The listing builds one solid part. Answer for the finished solid, in the listing's coordinates (mm). Face numbers are marked on the shaded views. A direction names the side the tool comes from. Give positions to 0.01 mm unless a question says otherwise; leave off trailing zeros. Write each loop counter-clockwise with the first axis right and the second up, starting at its lowest first coordinate (ties: lowest second). Pieces come first, ordered by that corner, then holes.
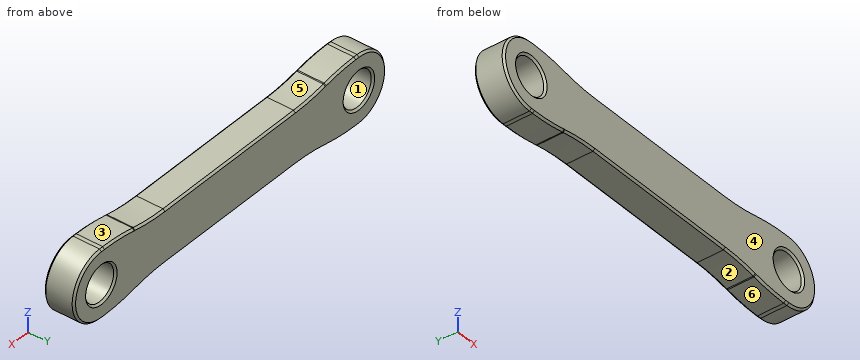
```python
from build123d import *

# Parameters (mm, degrees)
SKETCH1_R           = 4.7
BOSS_EXTRUDE1_DEPTH = 8
FILLET1_R           = 50
FILLET2_R           = 50
CHAMFER1_SIZE       = 0.5
CHAMFER2_SIZE       = 0.5


with BuildPart() as part:
    # Sketch1 → Boss-Extrude1 (new body)
    with BuildSketch(Plane(origin=(0, 0, 0), x_dir=(1, 0, 0), z_dir=(0, 1, 0))):
        with BuildLine():
            Line((6, 9), (16, 7))
            Line((16, 7), (69, 7))
            Line((69, 7), (79, 9))
            Line((79, 9), (85, 9))
            ThreePointArc((85, 9), (94, 0), (85, -9))
            Line((85, -9), (79, -9))
            Line((79, -9), (69, -7))
            Line((69, -7), (16, -7))
            Line((16, -7), (6, -9))
            Line((6, -9), (0, -9))
            ThreePointArc((0, -9), (-9, 0), (0, 9))
            Line((0, 9), (6, 9))
        make_face()
        with Locations(Location((0, 0, 0), (0, 0, 270))):
            Circle(SKETCH1_R, mode=Mode.SUBTRACT)
        with Locations(Location((85, 0, 0), (0, 0, 270))):
            Circle(SKETCH1_R, mode=Mode.SUBTRACT)
    extrude(amount=BOSS_EXTRUDE1_DEPTH)

    # Fillet1
    fillet1_edges = [part.edges().sort_by_distance(p)[0] for p in [
        (16, 4, -7),
        (69, 4, -7),
        (69, 4, 7),
        (16, 4, 7),
    ]]
    fillet(fillet1_edges, radius=FILLET1_R)

    # Fillet2
    fillet2_edges = [part.edges().sort_by_distance(p)[0] for p in [
        (6, 4, 9),
        (6, 4, -9),
        (79, 4, -9),
        (79, 4, 9),
    ]]
    fillet(fillet2_edges, radius=FILLET2_R)

    # Chamfer1
    chamfer1_edges = [part.edges().sort_by_distance(p)[0] for p in [
        (0, 0, -4.7),
        (0, 8, -4.7),
        (85, 0, -4.7),
        (85, 8, -4.7),
    ]]
    chamfer(chamfer1_edges, length=CHAMFER1_SIZE)

    # Chamfer2
    chamfer2_edges = [part.edges().sort_by_distance(p)[0] for p in [
        (0.52451216, 0, 9),
        (-9, 0, 0),
        (84.47548784, 0, -9),
        (94, 0, 0),
        (94, 8, 0),
        (84.47548784, 8, -9),
        (74, 0, 8),
        (-9, 8, 0),
        (74, 8, 8),
        (42.5, 0, 7),
        (42.5, 8, 7),
        (0.52451216, 8, 9),
        (42.5, 0, -7),
        (42.5, 8, -7),
        (11, 0, -8),
        (11, 8, -8),
        (68.975905219, 0, 7.243333667),
        (68.975905219, 8, 7.243333667),
        (16.024094781, 0, 7.243333667),
        (16.024094781, 8, 7.243333667),
        (68.975905219, 0, -7.243333667),
        (68.975905219, 8, -7.243333667),
        (16.024094781, 0, -7.243333667),
        (16.024094781, 8, -7.243333667),
        (74, 0, -8),
        (74, 8, -8),
        (11, 0, 8),
        (0.52451216, 0, -9),
        (84.47548784, 0, 9),
        (5.975905219, 0, 8.756666333),
        (79.024094781, 0, 8.756666333),
        (5.975905219, 0, -8.756666333),
        (79.024094781, 0, -8.756666333),
        (11, 8, 8),
        (84.47548784, 8, 9),
        (0.52451216, 8, -9),
        (5.975905219, 8, 8.756666333),
        (79.024094781, 8, 8.756666333),
        (5.975905219, 8, -8.756666333),
        (79.024094781, 8, -8.756666333),
    ]]
    chamfer(chamfer2_edges, length=CHAMFER2_SIZE)


solid = part.part
```
Item 1: A cutting plane is placed at C-C, the plane x = 53. Give the vertices of the cut face in (y, z).
Conclusion:
outline: (0, -6.5) - (0.5, -7) - (7.5, -7) - (8, -6.5) - (8, 6.5) - (7.5, 7) - (0.5, 7) - (0, 6.5) - close
Item 2: Each of these flat-tipped pins is pushed along its axis until it touches: P1, Ø2, axis at x = 77.5, y = 6.5, coming from the +Z side; P2, Ø3.5, axis at x = 42.5, y = 3, coming from the -Z side; P3, Ø4, axis at x = 18, y = 3, coming from the -Z side; P4, Ø1, axis at x = 1.5, z = 2, coming from the +Y side. Where does it stop, or does it pass through?
Conclusion:
P1: stops at z = 8.7
P2: stops at z = -7
P3: stops at z = -7.25
P4: passes through
Item 3: A cutting plane is placed at A-A, the plane z = 0. Give the vertices of the cut face in (x, y).
Conclusion:
outline: (-9, 0.5) - (-8.5, 0) - (-5.2, 0) - (-4.7, 0.5) - (-4.7, 7.5) - (-5.2, 8) - (-8.5, 8) - (-9, 7.5) - close; (4.7, 0.5) - (5.2, 0) - (79.8, 0) - (80.3, 0.5) - (80.3, 7.5) - (79.8, 8) - (5.2, 8) - (4.7, 7.5) - close; (89.7, 0.5) - (90.2, 0) - (93.5, 0) - (94, 0.5) - (94, 7.5) - (93.5, 8) - (90.2, 8) - (89.7, 7.5) - close
Item 4: Determine the mould class of the marked faces 1, 2 and 3 for opening direction Z: pulls with the +Z half, pulls with the -Z half, needs draft (parallel to the pull), parting line crosses it, or undercut.
Conclusion:
face 1: undercut
face 2: pulls with the -Z half
face 3: pulls with the +Z half
Item 5: A cutting plane is placed at B-B, the plane y = 6.25. Give the vertices of the cut face in (x, z).
Conclusion:
outline: (0, -9) - (1.05, -9) arc R50 ccw to (10.85, -8.03) - (11.15, -7.97) arc R50 cw to (20.95, -7) - (64.05, -7) arc R50 cw to (73.85, -7.97) - (74.15, -8.03) arc R50 ccw to (83.95, -9) - (85, -9) arc R9 ccw to (85, 9) - (83.95, 9) arc R50 ccw to (74.15, 8.03) - (73.85, 7.97) arc R50 cw to (64.05, 7) - (20.95, 7) arc R50 cw to (11.15, 7.97) - (10.85, 8.03) arc R50 ccw to (1.05, 9) - (0, 9) arc R9 ccw to start; hole circle Ø9.4 at (0, 0); hole circle Ø9.4 at (85, 0)
Item 6: Which of the six approach directions +Z, -Z, +X, -X, +Y, -Y give full straight-line access (tool end or side, diameter ignored) to the marked faces 4, 5 and 6?
Conclusion:
face 4: +Z, -Z, +X, -X, -Y
face 5: +Z, +Y, -Y
face 6: -Z, +Y, -Y
Item 7: Consider probe 1 along X at (y, z) = (2.25, 0); probe 2 along X at (y, z) = (3.5, -2.75); probe 3 along Z at (x, y) = (52.5, 6.25). Determine where each line is inside the solid, lowest interval first.
Conclusion:
probe 1: x = -9 to -4.7, 4.7 to 80.3, 89.7 to 94
probe 2: x = -8.57 to -3.81, 3.81 to 81.19, 88.81 to 93.57
probe 3: z = -7 to 7
